```python
from build123d import *

# Parameters (mm, degrees)
F0_W     = 2032
F0_H     = 76.2
F1_DEPTH = 76.2
F2_W     = 2032
F2_H     = 69.85
F3_DEPTH = 69.85
F5_DEPTH = 76.2


with BuildPart() as f1:
    # F0 (on Top) → F1 (new body)
    with BuildSketch(Plane.XY):
        with Locations((-1016, 38.1)):
            Rectangle(F0_W, F0_H)
    extrude(amount=-F1_DEPTH)

    # F2 (on face) → F3 (cut)
    with BuildSketch(Plane.XY):
        with Locations((-1016, 34.925)):
            Rectangle(F2_W, F2_H)
    extrude(amount=-F3_DEPTH, mode=Mode.SUBTRACT)

    # F4 (on face) → F5 (cut)
    with BuildSketch(Plane.XY):
        Polygon((-1955.8, 0), (-2032, 76.2), (-2032, 0), align=None)
        Polygon((0, 76.2), (-76.2, 0), (0, 0), align=None)
    extrude(amount=-F5_DEPTH, mode=Mode.SUBTRACT)


solid = f1.part
```
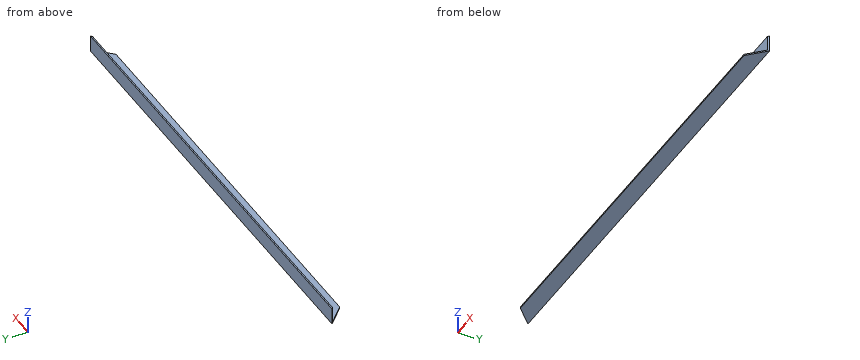
Part model, mm, in its own coordinate system. Round coordinates to 2 decimals unless told otherwise and drop trailing zeros. Write each loop counter-clockwise with the first axis right and the second up, starting at its lowest first coordinate (ties: lowest second). Pieces come first, ordered by that corner, then holes. Notation, with made-up numbers: (4.25, 32.5) -> (23.25, 32.5) arc R27 cw to (23.25, 51.5) -> close; hole circle Ø10 at (-7, 71). An arc over 180 degrees is marked (long way). Return JSON: item names as keys, results as strings. Group by question number.
Q1. Probe L1, parallel to Y at x = -1847, z = -31; L2, parallel to Z at x = -630, y = 61; L3, parallel to X at y = 70.5, z = -68.5. List the from-to ranges inside material, lowest first. Write a range as [from, to].
Q2. Saw through at B-B on x = -1802. Write the cut outline in (y, z).
Q3. Saw through at C-C on z = -42. Write the cut outline in (x, y).
Q4. Saw through at A-A on y = 49.5. Write the cut outline in (x, z).
Q5. Pin check, flat tips, straight feed: pin 1 (1.5 mm diameter, centred on x = -547.5, y = 41, fed in from +Z); pin 2 (4 mm diameter, centred on y = 68, z = -44.5, fed in from -X); pin 3 (4 mm diameter, centred on y = 68.5, z = -30, fed in from -X). Stop position of each tip, or through.
Answer:
{
 "1": {"L1": "[69.85, 76.2]", "L2": "[-76.2, -69.85]", "L3": "[-2026.3, -5.7]"},
 "2": {"outline": "(0, -76.2) -> (76.2, -76.2) -> (76.2, 0) -> (69.85, 0) -> (69.85, -69.85) -> (0, -69.85) -> close"},
 "3": {"outline": "(-2032, 76.2) -> (-2025.65, 69.85) -> (-6.35, 69.85) -> (0, 76.2) -> close"},
 "4": {"outline": "(-2005.3, -76.2) -> (-26.7, -76.2) -> (-26.7, -69.85) -> (-2005.3, -69.85) -> close"},
 "5": {"pin 1": "z = -69.85", "pin 2": "x = -2025.8", "pin 3": "x = -2026.3"}
}
